Read the model definition and answer for the solid it produces. Units are mm, in the model's axes. A direction names the side the tool comes from. Give positions to 0.01 mm unless a question says otherwise; leave off trailing zeros. One line per item, written item: value.
from build123d import *

# Parameters (mm, degrees)
BOX001_W     = 100
BOX001_H     = 120
BOX001_DEPTH = 600


with BuildPart() as cube001:
    # Box001 → Box001 (new body)
    with BuildSketch(Plane(origin=(4805, -60, -110), x_dir=(1, 0, 0), z_dir=(0, 0, 1))):
        with Locations((50, 60)):
            Rectangle(BOX001_W, BOX001_H)
    extrude(amount=BOX001_DEPTH)


with BuildPart() as sweep002:
    # Sweep002: sweep along a path in Sketch005
    with BuildLine(Plane.XZ) as sweep002_path:
        Line((4901.525879, 0.31053), (3518.000977, 0.31053))
    # Sketch004 → Sweep002 (sweep)
    with BuildSketch(Plane.YZ.offset(4700)):
        with BuildLine():
            add(Edge.make_bspline(
                [(0, 573.341003), (-451.187195, 557.981873), (-571.498, 209.848953), (-571.498, 209.848953)],
                knots=[0, 0, 0, 0, 1, 1, 1, 1], degree=3))
            Line((-571.498, 209.848953), (-571.498, -197.16))
            add(Edge.make_bspline(
                [(-571.498, -197.16), (-276.684204, -306.229828), (0, -304.212738)],
                knots=[0, 0, 0, 1, 1, 1], degree=2))
            Line((0, -304.212738), (0, 573.341003))
        make_face()
    sweep(path=sweep002_path.line)


with BuildPart() as cut001:
    # Part__Mirroring004: instance of Sweep002
    add(sweep002.part.mirror(Plane(origin=(0, 0, 0), x_dir=(1, 0, 0), z_dir=(0, 1, 0))))

    # Fusion: union Sweep002
    add(sweep002.part)

    # Cut001: cut Cube001
    add(cube001.part, mode=Mode.SUBTRACT)


solid = cut001.part
1) Which of the six approach directions +Z, -Z, +X, -X, +Y, -Y give full straight-line access (tool end or side, diameter ignored) to faces 3 (the face through (4200, -571.498, 9)), 4 (the face through (4805, -1, 186))?
Reported:
face 3: +Z, -Z, +X, -X, -Y
face 4: +X
2) Determine the mould class of faces 1 (the face through (4901.526, 119, 127)), 2 (the face through (4853, 60, 186)) for opening direction Z: +Z half, -Z half, draft (parallel to the pull), parting line (faces both ways), or undercut.
Reported:
face 1: draft
face 2: undercut
3) Consider probe 1 along Y at (x, z) = (4808, 138.5); probe 2 along Y at (x, z) = (3749, 308); probe 3 along Y at (x, z) = (4581.5, 354). Determine where each line is inside the solid, lowest interval first.
Reported:
probe 1: y = -571.5 to -60, 60 to 571.5
probe 2: y = -518.66 to 518.66
probe 3: y = -483.72 to 483.72
4) Each of these flat-tipped pins is pushed along its axis until it touches: pin 1 Ø3 at (x, z) = (3810, 438) entering from -Y; pin 2 Ø8 at (x, y) = (4081, 443) entering from +Z; pin 3 Ø4 at (x, z) = (4753, 365.5) entering from -Y. Where does it stop, or does it pass through?
Reported:
pin 1: stops at y = -398.94
pin 2: stops at z = 401.62
pin 3: stops at y = -475.57
